Part model, mm, in its own coordinate system. Face numbers are marked on the shaded views. A direction names the side the tool comes from. Round coordinates to 2 decimals unless told otherwise and drop trailing zeros. Loops run counter-clockwise (first coordinate to the right, second up) from the corner with the lowest first, then second, coordinate; pieces in that order, holes last. Notation, with made-up numbers: (9, 72.25) - (32, 72.25) arc R7 ccw to (32, 80.25) - close; hole circle Ø3 at (-34, 62.5). An arc over 180 degrees is marked (long way). Put each result on its own line as item: value.
from build123d import *

# Parameters (mm, degrees)
SKETCH1_R            = 43.5
BOSS_EXTRUDE1_DEPTH  = 4.7498
SKETCH2_R            = 31
SKETCH2_R_2          = 16.5
CUT_EXTRUDE1_DEPTH   = 21.73
BOSS_EXTRUDE2_DEPTH  = 4.7498
CIRPATTERN1_COUNT    = 3
FILLET1_R            = 5
M4_CLEARANCE_HOLE1_D = 4.8


with BuildPart() as part:
    # Sketch1 → Boss-Extrude1 (new body)
    with BuildSketch(Plane.XY):
        Circle(SKETCH1_R)
    extrude(amount=BOSS_EXTRUDE1_DEPTH)

    # Sketch2 → Cut-Extrude1 (cut)
    with BuildSketch(Plane.XY.offset(4.7498)):
        Circle(SKETCH2_R)
        Circle(SKETCH2_R_2, mode=Mode.SUBTRACT)
    extrude(amount=-CUT_EXTRUDE1_DEPTH, mode=Mode.SUBTRACT)

    # Sketch3 → Boss-Extrude2 (add)
    with BuildSketch(Plane.XY.offset(4.7498)):
        with BuildLine():
            Line((-3, 16.22498074), (-3, 30.854497241))
            ThreePointArc((-3, 30.854497241), (0, 31), (3, 30.854497241))
            Line((3, 30.854497241), (3, 16.22498074))
            ThreePointArc((3, 16.22498074), (0, 16.5), (-3, 16.22498074))
        make_face()
    boss_extrude2 = extrude(amount=-BOSS_EXTRUDE2_DEPTH)

    # CirPattern1: Boss-Extrude2 ×3 about axis
    cirpattern1_axis = Axis((0, 0, 0), (0, 0, 1))
    for i in range(1, CIRPATTERN1_COUNT):
        add(boss_extrude2.rotate(cirpattern1_axis, i * 360 / CIRPATTERN1_COUNT))

    # Fillet1
    fillet1_edges = [part.edges().sort_by_distance(p)[0] for p in [
        (-15.551245496, -5.514414158, 2.3749),
        (-12.551245496, -10.710566581, 2.3749),
        (-25.220778432, -18.025324832, 2.3749),
        (-28.220778432, -12.829172409, 2.3749),
        (12.551245496, -10.710566581, 2.3749),
        (15.551245496, -5.514414158, 2.3749),
        (28.220778432, -12.829172409, 2.3749),
        (25.220778432, -18.025324832, 2.3749),
        (3, 16.22498074, 2.3749),
        (-3, 16.22498074, 2.3749),
        (-3, 30.854497241, 2.3749),
        (3, 30.854497241, 2.3749),
    ]]
    fillet(fillet1_edges, radius=FILLET1_R)

    # M4 Clearance Hole1 (through all)
    with Locations(Plane.XY.offset(4.7498)):
        with Locations((-8, 8), (-8, -8), (8, -8), (8, 8)):
            Hole(M4_CLEARANCE_HOLE1_D / 2)


solid = part.part
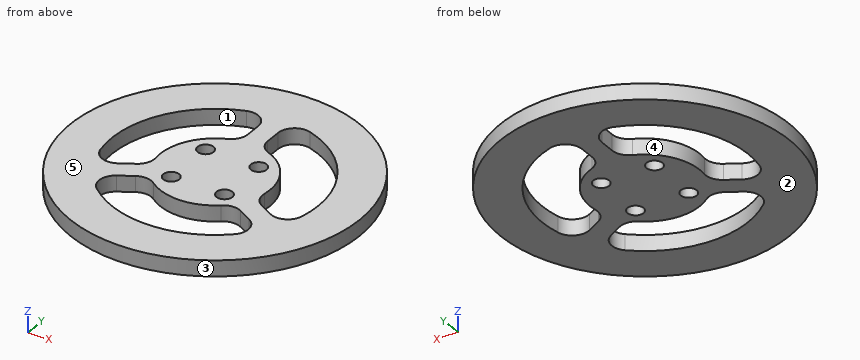
1. Band-saw the part on D-D (x = -27.5). List the corners of the cut face in (y, z), plus the area to 3 significant figures.
A:
outline: (-33.7, 0) - (-9.99, 0) - (-9.99, 4.75) - (-33.7, 4.75) - close; (14.31, 0) - (33.7, 0) - (33.7, 4.75) - (14.31, 4.75) - close
area: 205 mm²
2. Band-saw the part on A-A (y = 0). List the corners of the cut face in (x, z).
A:
outline: (-43.5, 0) - (-31, 0) - (-31, 4.75) - (-43.5, 4.75) - close; (-16.5, 0) - (16.5, 0) - (16.5, 4.75) - (-16.5, 4.75) - close; (31, 0) - (43.5, 0) - (43.5, 4.75) - (31, 4.75) - close
3. Probe line 1 along X through (y, z) = (12, 2.2); line 2 along Y through (x, z) = (-8, 1.6); line 3 along Y through (x, z) = (14, 2.2). List the from-to ranges inside material, lowest first. Write a range as [from, to].
A:
line 1: x = [-41.81, -28.58], [-11.32, 11.32], [28.58, 41.81]
line 2: y = [-42.76, -29.95], [-14.43, -10.4], [-5.6, 5.6], [10.4, 14.43], [29.74, 42.76]
line 3: y = [-41.19, -27.66], [-11.96, 8.73], [27.66, 41.19]
4. Two-plate mould, pull along Y, no slides. Class the marked faces 1, 2 and 3: pulls with the +Y half, pulls with the -Y half, needs draft (parallel to the pull), parting line crosses it, or undercut.
A:
face 1: undercut
face 2: needs draft
face 3: parting line crosses it
5. Pin check, flat tips, straight feed: P1, Ø4, axis at x = 8, y = -8, coming from the -Z side; P2, Ø2, axis at x = -26, z = 0.5, coming from the -Y side; P3, Ø2.5, axis at y = 21.5, z = 2, coming from the -X side; P4, Ø1, axis at y = -13, z = 0.5, coming from the -X side. Stop position of each tip, or through.
A:
P1: passes through
P2: stops at y = -35.6
P3: stops at x = -38.5
P4: stops at x = -41.67
6. Tool access for the marked faces 4 and 5: list every direction of +Z, -Z, +X, -X, +Y, -Y with a clear straight run to the whole face (end or side of a thin tool).
A:
face 4: +Z, -Z
face 5: +Z, +X, -X, +Y, -Y
7. Band-saw the part on C-C (z = 2.9). Give the number of separate pieces and of enclosed holes in the cut face, plus the area to 3 significant figures.
A:
separate pieces: 1
enclosed holes: 7
area: 4,040 mm²
8. Band-saw the part on B-B (x = 0). List the corners of the cut face in (y, z).
A:
outline: (-43.5, 0) - (-31, 0) - (-31, 4.75) - (-43.5, 4.75) - close; (-16.5, 0) - (43.5, 0) - (43.5, 4.75) - (-16.5, 4.75) - close
